Here's how the part is built. I have some questions about the finished solid (model axes, mm). Round coordinates to 2 decimals unless told otherwise and drop trailing zeros. Loops run counter-clockwise (first coordinate to the right, second up) from the corner with the lowest first, then second, coordinate; pieces in that order, holes last. Notation, with made-up numbers: (73.25, 56) -> (103.25, 56) arc R13 ccw to (103.25, 76) -> close; hole circle Ø11 at (10.25, -38.75). An arc over 180 degrees is marked (long way). Use one line per item in the form item = value. Start each with the question number.
Item 1: Thinking about a two-plate mould opening in X: for faces 1 (the face through (-41.955, -23.766, 1.565)), 2 (the face through (3.1, 14.1, 3.175)), which applies, released by +X, released by -X, zero draft, split by the parting line, or undercut?
Item 2: I'm going to push flat-ended pins straight in: pin 1 Ø1.5 at (x, z) = (7.5, 1.5) entering from -Y; pin 2 Ø15 at (x, y) = (-27.5, -15.88) entering from -Z. Where does each tip first touch, or does it pass through?
Item 3: If we section it at C-C (z = 1.5): State how many separate pieces and enclosed holes the cut face has, then the cut area to 3 significant figures.
Item 4: If we section it at B-B (x = -38): Write out the boundary of the cut face in (y, z) (3 decimals).
Item 5: If I drill on L1, parallel to X at y = -16, z = 2.75; L2, parallel to Y at x = 4, z = 0.25; L3, parallel to X at y = -18, z = 2.8, over which ranges is the centre line in solid material (lowest first)? Write a range as [from, to].
Item 6: If we section it at A-A (y = -10): Write out the boundary of the cut face in (x, z) (3 decimals).
```python
from build123d import *

# Parameters (mm, degrees)
F1_DEPTH = 3.175
F2_R     = 27.94


with BuildPart() as f1:
    # F0 (on Top) → F1 (new body)
    with BuildSketch(Plane.XY):
        with BuildLine():
            ThreePointArc((11.3701248677, 19.83178914), (6.1240473604, 16.4588413278), (0, 15.2781))
            ThreePointArc((0, 15.2781), (-6.1240473604, 16.4588413278), (-11.3701248677, 19.83178914))
            ThreePointArc((-11.3701248677, 19.83178914), (-19.7973407305, 11.43), (-22.8598956316, -0.0690775904))
            ThreePointArc((-22.8598956316, -0.0690775904), (-14.3112015848, -6.0019814071), (-11.0244065702, -15.875))
            ThreePointArc((-11.0244065702, -15.875), (-11.1411614048, -17.8327324208), (-11.4897707639, -19.7627115496))
            ThreePointArc((-11.4897707639, -19.7627115496), (0, -22.86), (11.4897707639, -19.7627115496))
            ThreePointArc((11.4897707639, -19.7627115496), (13.2312227216, -7.63905), (22.8598956316, -0.0690775904))
            ThreePointArc((22.8598956316, -0.0690775904), (22.8599739079, -0.0345388346), (22.86, 0))
            ThreePointArc((22.86, 0), (19.7800487168, 11.4598984621), (11.3701248677, 19.83178914))
        make_face()
        with BuildLine():
            ThreePointArc((14.2494, 0), (-10.0758473678, -10.0758473678), (0, 14.2494))
            ThreePointArc((0, 14.2494), (10.0758473678, 10.0758473678), (14.2494, 0))
        make_face(mode=Mode.SUBTRACT)
        with BuildLine():
            ThreePointArc((-11.3701248677, 19.83178914), (-6.1240473604, 16.4588413278), (0, 15.2781))
            Line((0, 15.2781), (0, 19.0881))
            ThreePointArc((0, 19.0881), (-3.9717674438, 19.7271561192), (-7.5426183918, 21.57981714))
            ThreePointArc((-7.5426183918, 21.57981714), (-9.4966765172, 20.7940552834), (-11.3701248677, 19.83178914))
        make_face()
        with BuildLine():
            Line((0, 19.0881), (0, 15.2781))
            ThreePointArc((0, 15.2781), (6.1240473604, 16.4588413278), (11.3701248677, 19.83178914))
            ThreePointArc((11.3701248677, 19.83178914), (9.4966765172, 20.7940552834), (7.5426183918, 21.57981714))
            ThreePointArc((7.5426183918, 21.57981714), (3.9717674438, 19.7271561192), (0, 19.0881))
        make_face()
        with BuildLine():
            ThreePointArc((16.4719, 31.75), (-6.4821265724, 46.8928374061), (-11.3701248677, 19.83178914))
            ThreePointArc((-11.3701248677, 19.83178914), (-9.4966765172, 20.7940552834), (-7.5426183918, 21.57981714))
            ThreePointArc((-7.5426183918, 21.57981714), (-5.6929707445, 43.0598981301), (12.6619, 31.75))
            ThreePointArc((12.6619, 31.75), (11.3098981301, 26.0570292555), (7.5426183918, 21.57981714))
            ThreePointArc((7.5426183918, 21.57981714), (9.4966765172, 20.7940552834), (11.3701248677, 19.83178914))
            ThreePointArc((11.3701248677, 19.83178914), (15.1428374061, 25.2678734276), (16.4719, 31.75))
        make_face()
        with BuildLine():
            ThreePointArc((-22.4599790482, -4.2578094317), (-22.7565183817, -2.1726645263), (-22.8598956316, -0.0690775904))
            ThreePointArc((-22.8598956316, -0.0690775904), (-41.7613904188, -24.11095), (-11.4897707639, -19.7627115496))
            ThreePointArc((-11.4897707639, -19.7627115496), (-13.2598418645, -18.6213907571), (-14.9173606564, -17.3220077083))
            ThreePointArc((-14.9173606564, -17.3220077083), (-38.4618336303, -22.20595), (-22.4599790482, -4.2578094317))
        make_face()
        with BuildLine():
            ThreePointArc((-11.0244065702, -15.875), (-14.3112015848, -6.0019814071), (-22.8598956316, -0.0690775904))
            ThreePointArc((-22.8598956316, -0.0690775904), (-22.7565183817, -2.1726645263), (-22.4599790482, -4.2578094317))
            ThreePointArc((-22.4599790482, -4.2578094317), (-16.9111002174, -8.9268262774), (-14.8344065702, -15.875))
            ThreePointArc((-14.8344065702, -15.875), (-14.8551621031, -16.5996917773), (-14.9173606564, -17.3220077083))
            ThreePointArc((-14.9173606564, -17.3220077083), (-13.2598418645, -18.6213907571), (-11.4897707639, -19.7627115496))
            ThreePointArc((-11.4897707639, -19.7627115496), (-11.1411614048, -17.8327324208), (-11.0244065702, -15.875))
        make_face()
        with BuildLine():
            ThreePointArc((22.4599790482, -4.2578094317), (22.7565183817, -2.1726645263), (22.8598956316, -0.0690775904))
            ThreePointArc((22.8598956316, -0.0690775904), (13.2312227216, -7.63905), (11.4897707639, -19.7627115496))
            ThreePointArc((11.4897707639, -19.7627115496), (13.2598418645, -18.6213907571), (14.9173606564, -17.3220077083))
            ThreePointArc((14.9173606564, -17.3220077083), (16.53077951, -9.54405), (22.4599790482, -4.2578094317))
        make_face()
        with BuildLine():
            ThreePointArc((43.9682065702, -15.875), (37.369325163, -2.6898950147), (22.8598956316, -0.0690775904))
            ThreePointArc((22.8598956316, -0.0690775904), (22.7565183817, -2.1726645263), (22.4599790482, -4.2578094317))
            ThreePointArc((22.4599790482, -4.2578094317), (34.4444802928, -5.2897936472), (40.1582065702, -15.875))
            ThreePointArc((40.1582065702, -15.875), (28.2209983475, -28.5161444671), (14.9173606564, -17.3220077083))
            ThreePointArc((14.9173606564, -17.3220077083), (13.2598418645, -18.6213907571), (11.4897707639, -19.7627115496))
            ThreePointArc((11.4897707639, -19.7627115496), (29.454038991, -32.2301451653), (43.9682065702, -15.875))
        make_face()
    extrude(amount=F1_DEPTH)

    # F2
    f2_edges = [f1.edges().sort_by_distance(p)[0] for p in [
        (-11.370125, 19.831789, 1.5875),
        (-22.859896, -0.069078, 1.5875),
        (-11.489771, -19.762712, 1.5875),
        (22.859896, -0.069078, 1.5875),
        (11.489771, -19.762712, 1.5875),
        (11.370125, 19.831789, 1.5875),
    ]]
    fillet(f2_edges, radius=F2_R)


solid = f1.part
```
Values found:
q1.face_1 = undercut
q1.face_2 = zero draft
q2.pin_1 = -24.09
q2.pin_2 = through
q3.separate_pieces = 1
q3.enclosed_holes = 4
q3.area = 1,870 mm2
q4.outline = (-28.563, 0) -> (-22.946, 0) -> (-22.946, 3.175) -> (-28.563, 3.175) -> close; (-8.804, 0) -> (-3.187, 0) -> (-3.187, 3.175) -> (-8.804, 3.175) -> close
q5.L1 = [-43.97, -40.16], [-14.84, 14.84], [40.16, 43.97]
q5.L2 = [-23.14, -13.68], [13.68, 19.74], [43.76, 47.73]
q5.L3 = [-43.83, -39.98], [-15.01, 15.01], [39.98, 43.83]
q6.outline = (-42.885, 0) -> (-38.713, 0) -> (-38.713, 3.175) -> (-42.885, 3.175) -> close; (-16.28, 0) -> (-10.151, 0) -> (-10.151, 3.175) -> (-16.28, 3.175) -> close; (10.151, 0) -> (16.28, 0) -> (16.28, 3.175) -> (10.151, 3.175) -> close; (38.713, 0) -> (42.885, 0) -> (42.885, 3.175) -> (38.713, 3.175) -> close
